```python
from build123d import *

# Parameters (mm, degrees)
F0_R           = 11
F1_DEPTH       = 8
F3_R           = 11.4612754368
F3_R_2         = 5
F4_DEPTH       = 9
F6_D           = 5
F6_CBORE_D     = 10
F6_CBORE_DEPTH = 4
F7_R           = 1.99999


# Not quite as in the source:
# - a fillet or chamfer is up to 0.001 mm smaller than in the source, because OpenCascade refuses the exact size


with BuildPart() as f1:
    # F0 (on Front) → F1 (new body, symmetric)
    with BuildSketch(Plane.XZ):
        with BuildLine():
            Line((16, 8), (16, 30.7))
            ThreePointArc((16, 30.7), (0, 46.7), (-16, 30.7))
            Line((-16, 30.7), (-16, 8))
            Line((-16, 8), (-30, 8))
            Line((-30, 8), (-30, 0))
            Line((-30, 0), (30, 0))
            Line((30, 0), (30, 8))
            Line((30, 8), (16, 8))
        make_face()
        with Locations((0, 30.7)):
            Circle(F0_R, mode=Mode.SUBTRACT)
    extrude(amount=F1_DEPTH, both=True)

    # F3 (on offset) → F4 (join)
    with BuildSketch(Plane.XZ.offset(1)):
        with Locations((0, 30.7003352791)):
            Circle(F3_R)
        with Locations((0, 30.7003352791)):
            Circle(F3_R_2, mode=Mode.SUBTRACT)
    extrude(amount=-F4_DEPTH)

    # F6 (through all)
    with Locations(Plane.XY.offset(8)):
        with Locations((-23, 0), (23, 0)):
            CounterBoreHole(F6_D / 2, F6_CBORE_D / 2, F6_CBORE_DEPTH)

    # F7 (radius 2 in the source; OpenCascade refuses exactly that, so slightly less here)
    f7_edges = [f1.edges().sort_by_distance(p)[0] for p in [
        (-30, -8, 4),
        (-23, -8, 8),
        (-16, -8, 19.35),
        (23, -8, 8),
        (30, -8, 4),
        (-30, 0, 8),
        (30, 0, 8),
    ]]
    fillet(f7_edges, radius=F7_R)


solid = f1.part
```
Input: part model. Units: mm. Frame: model coordinates. A direction names the side the tool comes from. Coordinates: 2 decimals unless noted, no trailing zeros. Loops run counter-clockwise (first coordinate to the right, second up) from the corner with the lowest first, then second, coordinate; pieces in that order, holes last.
Q1. Section D-D, the plane x = 0. Return the cut outline in (y, z), and give its area (3 significant figures).
Results are:
outline: (-8, 0) - (8, 0) - (8, 25.7) - (-1, 25.7) - (-1, 19.7) - (-8, 19.7) - close; (-8, 41.7) - (-1, 41.7) - (-1, 35.7) - (8, 35.7) - (8, 46.7) - (-6, 46.7) arc R2 ccw to (-8, 44.7) - close
area: 502 mm2
Q2. Section B-B, the plane y = 1.75. Return the cut outline in (x, z).
Results are:
outline: (-30, 0) - (-24.79, 0) - (-24.79, 4) - (-27.68, 4) - (-27.68, 8) - (-28, 8) arc R2 ccw to (-30, 6) - close; (-21.21, 0) - (21.21, 0) - (21.21, 4) - (18.32, 4) - (18.32, 8) - (16, 8) - (16, 30.7) arc R16 ccw to (-16, 30.7) - (-16, 8) - (-18.32, 8) - (-18.32, 4) - (-21.21, 4) - close; (24.79, 0) - (30, 0) - (30, 6) arc R2 ccw to (28, 8) - (27.68, 8) - (27.68, 4) - (24.79, 4) - close; hole circle Ø10 at (0, 30.7)
Q3. Section C-C, the plane z = 15.5. Return the cut outline in (x, y), and give its area (3 significant figures).
Results are:
outline: (-16, -6) arc R2 ccw to (-14, -8) - (14, -8) arc R2 ccw to (16, -6) - (16, 8) - (-16, 8) - close
area: 510 mm2
Q4. Mould query, pull axis X, two halves, no side actions, for faces 4 (the flat face through (0, -8, 18)), 5 (the flat face through (2.3, -1, 26)), 6 (the flat face through (30, 1, 3)), 7 (the cylindrical face through (-28, 0, 6)). Classes: +X half, -X half, draft (parallel to the pull), parting line (faces both ways), or undercut.
Results are:
face 4: draft
face 5: undercut
face 6: +X half
face 7: undercut
Q5. Contact query for flat-ended pins moving along their axis: pin 1 (6.5 mm diameter, centred on x = 23, y = 0, fed in from -Z); pin 2 (4 mm diameter, centred on y = -5, z = 19, fed in from +X); pin 3 (5 mm diameter, centred on x = 23, y = -2, fed in from +Z); pin 4 (5 mm diameter, centred on x = -21, y = -5.5, fed in from +Z). Output: stop coordinate, or through.
Results are:
pin 1: stops at z = 0
pin 2: stops at x = 16
pin 3: stops at z = 4
pin 4: stops at z = 8
Q6. Section A-A, the plane x = -23. Return the cut outline in (y, z), and give its area (3 significant figures).
Results are:
outline: (-8, 0) - (-2.5, 0) - (-2.5, 4) - (-5, 4) - (-5, 8) - (-6, 8) arc R2 ccw to (-8, 6) - close; (2.5, 0) - (8, 0) - (8, 8) - (5, 8) - (5, 4) - (2.5, 4) - close
area: 67.1 mm2
Q7. Line query: line 1 along Z through (x, y) = (0, 1.25); line 2 along Y through (x, z) = (23, 5); line 3 along X through (y, z) = (-0.25, 31). Output: solid intervals per line, ascending.
Results are:
line 1: z = 0 to 25.7, 35.7 to 46.7
line 2: y = -8 to -5, 5 to 8
line 3: x = -16 to -4.99, 4.99 to 16
Q8. Set-up query: faces 1 (the cylindrical face through (20.9, -7.4, 7.43)), 2 (the cylindrical face through (18, 0, 6)), 3 (the flat face through (16, 1, 19)). Return all of +Z, -Z, +X, -X, +Y, -Y with unobstructed straight access to the full face (end or side cutting, diameter ignored); none if empty.
Results are:
face 1: +Z, +X, -Y
face 2: +Z
face 3: +Z, +X, +Y, -Y
